Build history of the part. All positions in model axes, mm. Face numbers are marked on the shaded views. A direction names the side the tool comes from. Round coordinates to 2 decimals unless told otherwise and drop trailing zeros. Order: outer loops, then holes, each group sorted by start corner. A loop starts at its lowest first (then second) coordinate and runs counter-clockwise, first axis right, second up. Notation, with made-up numbers: (34.5, -13.75) -> (46.5, -13.75) arc R6 cw to (46.5, -3.75) -> close; hole circle Ø5 at (85.5, 25.25). An arc over 180 degrees is marked (long way). Answer as a JSON object with one key per item and string values.
from build123d import *

# Parameters (mm, degrees)
BRIDA_BASE1_DEPTH          = 89.15
CORTAR_EXTRUIR3_DEPTH      = 100.859660931
CORTAR_EXTRUIR3_DEPTH_BACK = 100.859660931
CROQUIS7_W                 = 3
CROQUIS7_H                 = 17.495
REDONDEO6_R                = 1
REDONDEO8_RADIUS           = 7.11
REDONDEO8_LENGTH           = 3.175
REDONDEO9_RADIUS           = 7.11
REDONDEO9_LENGTH           = 3.175
CORTAR_EXTRUIR4_DEPTH      = 100.859660931
CORTAR_EXTRUIR4_DEPTH_BACK = 100.859660931
CROQUIS14_R                = 1.5
CORTAR_EXTRUIR5_DEPTH      = 99.89399947
CORTAR_EXTRUIR5_DEPTH_BACK = 99.89399947
CROQUIS15_W                = 3.24
CROQUIS15_H                = 30.48


# Sheet-metal steps are written as plain solids
with BuildPart() as part:
    # Croquis1 → Brida base1 (new body)
    with BuildSketch(Plane.XY):
        with BuildLine():
            Line((25.4625, 0), (25.4625, 27.9034))
            ThreePointArc((25.4625, 27.9034), (25.246754855, 28.424254855), (24.7259, 28.64))
            Line((24.7259, 28.64), (0.7366, 28.64))
            ThreePointArc((0.7366, 28.64), (0.215745145, 28.424254855), (0, 27.9034))
            Line((0, 27.9034), (0, 0))
            Line((0, 0), (-3.175, 0))
            Line((-3.175, 0), (-3.175, 27.9034))
            ThreePointArc((-3.175, 27.9034), (-2.029318885, 30.669318885), (0.7366, 31.815))
            Line((0.7366, 31.815), (24.7259, 31.815))
            ThreePointArc((24.7259, 31.815), (27.491818885, 30.669318885), (28.6375, 27.9034))
            Line((28.6375, 27.9034), (28.6375, 0))
            Line((28.6375, 0), (25.4625, 0))
        make_face()
    extrude(amount=BRIDA_BASE1_DEPTH)

    # Croquis7 → Cortar-Extruir3 (cut, two sides: drawn at the far end of the back side and taken through both)
    with BuildSketch(Plane(origin=(28.6375, 0, 0), x_dir=(0, 0, -1), z_dir=(1, 0, 0)).offset(-CORTAR_EXTRUIR3_DEPTH_BACK)):
        with BuildLine():
            Line((0, 31.815), (-51.6, 31.815))
            Line((-51.6, 31.815), (-51.6, 18.22))
            ThreePointArc((-51.6, 18.22), (-50.428427125, 15.391572875), (-47.6, 14.22))
            Line((-47.6, 14.22), (0, 14.22))
            Line((0, 14.22), (0, 31.815))
        make_face()
        with Locations((-87.65, 8.7475)):
            Rectangle(CROQUIS7_W, CROQUIS7_H)
    extrude(amount=CORTAR_EXTRUIR3_DEPTH + CORTAR_EXTRUIR3_DEPTH_BACK, mode=Mode.SUBTRACT)

    # Redondeo6
    redondeo6_edges = [part.edges().sort_by_distance(p)[0] for p in [
        (-1.5875, 17.495, 86.15),
        (-1.5875, 17.495, 89.15),
        (-1.5875, 0, 86.15),
        (27.05, 17.495, 86.15),
        (27.05, 0, 86.15),
        (27.05, 17.495, 89.15),
    ]]
    fillet(redondeo6_edges, radius=REDONDEO6_R)

    # Redondeo8: full round fillet: the end face becomes a half cylinder, R = half its width
    redondeo8_face = Plane((27.05, 7.11, 0), x_dir=(-1, 0, 0), z_dir=(0, 0, -1))  # on the end face: x along it, z out of the body
    redondeo8_slab = redondeo8_face.offset(-REDONDEO8_RADIUS / 2) * Box(REDONDEO8_LENGTH, 2 * REDONDEO8_RADIUS, REDONDEO8_RADIUS, mode=Mode.PRIVATE)  # the body's end, R deep
    redondeo8_round = Plane((27.05, 7.11, 7.11), x_dir=(0, 0, -1), z_dir=(-1, 0, 0)) * Cylinder(REDONDEO8_RADIUS, REDONDEO8_LENGTH, mode=Mode.PRIVATE)  # its axis R under the face
    add(redondeo8_slab - redondeo8_round, mode=Mode.SUBTRACT)

    # Redondeo9: full round fillet: the end face becomes a half cylinder, R = half its width
    redondeo9_face = Plane((-1.5875, 7.11, 0), x_dir=(-1, 0, 0), z_dir=(0, 0, -1))  # on the end face: x along it, z out of the body
    redondeo9_slab = redondeo9_face.offset(-REDONDEO9_RADIUS / 2) * Box(REDONDEO9_LENGTH, 2 * REDONDEO9_RADIUS, REDONDEO9_RADIUS, mode=Mode.PRIVATE)  # the body's end, R deep
    redondeo9_round = Plane((-1.5875, 7.11, 7.11), x_dir=(0, 0, -1), z_dir=(-1, 0, 0)) * Cylinder(REDONDEO9_RADIUS, REDONDEO9_LENGTH, mode=Mode.PRIVATE)  # its axis R under the face
    add(redondeo9_slab - redondeo9_round, mode=Mode.SUBTRACT)

    # Croquis14 → Cortar-Extruir4 (cut, two sides: drawn at the far end of the back side and taken through both)
    with BuildSketch(Plane(origin=(28.6375, 0, 0), x_dir=(0, 0, -1), z_dir=(1, 0, 0)).offset(-CORTAR_EXTRUIR4_DEPTH_BACK)):
        with Locations((-7.11, 7.11)):
            Circle(CROQUIS14_R)
    extrude(amount=CORTAR_EXTRUIR4_DEPTH + CORTAR_EXTRUIR4_DEPTH_BACK, mode=Mode.SUBTRACT)

    # Croquis15 → Cortar-Extruir5 (cut, two sides: drawn at the far end of the back side and taken through both)
    with BuildSketch(Plane(origin=(0, 31.815, 0), x_dir=(1, 0, 0), z_dir=(0, 1, 0)).offset(-CORTAR_EXTRUIR5_DEPTH_BACK)):
        with Locations((12.73125, -70.375)):
            Rectangle(CROQUIS15_W, CROQUIS15_H)
    extrude(amount=CORTAR_EXTRUIR5_DEPTH + CORTAR_EXTRUIR5_DEPTH_BACK, mode=Mode.SUBTRACT)


solid = part.part
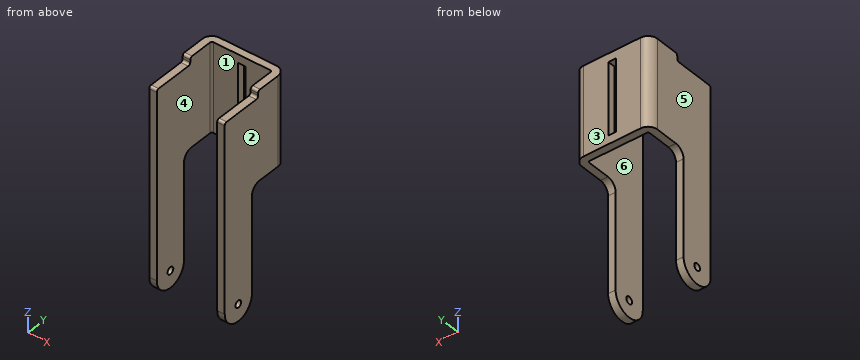
1) Cut at D-D, the plane x = 19. Give the cut face in (y, z) (3 decimals).
Checked values:
{"outline": "(28.64, 51.6) -> (31.815, 51.6) -> (31.815, 89.15) -> (28.64, 89.15) -> close"}
2) Cut at B-B, the plane z = 24. Give the cut face in (x, y) (1 decimal), plus the area to 3 significant figures.
Checked values:
{"outline": "(-3.2, 0) -> (0, 0) -> (0, 14.2) -> (-3.2, 14.2) -> close; (25.5, 0) -> (28.6, 0) -> (28.6, 14.2) -> (25.5, 14.2) -> close", "area": "90.3 mm²"}
3) Pull direction X, two halves, no side cores. Call the marked faces 1, 2, 3 and 4: pulls with the +X half, pulls with the -X half, needs draft (parallel to the pull), parting line crosses it, or undercut.
Checked values:
{"face 1": "undercut", "face 2": "pulls with the +X half", "face 3": "needs draft", "face 4": "undercut"}
4) Which spindle directions (+Z, -Z, +X, -X, +Y, -Y) get a long thin tool onto all of the face, cutting with end or side? Do the marked faces 5 and 6. Say none if no direction does.
Checked values:
{"face 5": "+Z, -Z, -X, +Y, -Y", "face 6": "+Z, -Z, -Y"}
5) Flat gauge pins, fed straight in: pin 1 Ø2.5 at (x, y) = (-1, 9) entering from +Z; pin 2 Ø1.6 at (y, z) = (30, 70) entering from -X; pin 3 Ø3.5 at (y, z) = (31, 72) entering from +X. Where does each tip first touch, or does it go through?
Checked values:
{"pin 1": "stops at z = 86.15", "pin 2": "stops at x = -2.95", "pin 3": "stops at x = 28.4"}
6) Probe L1, parallel to X at y = 20, z = 74 (1 decimal); L2, parallel to Y at x = -2.2, z = 7.11; L3, parallel to Z at x = 27, y = 7.11. List the from-to ranges inside material, lowest first. Write a range as from..to.
Checked values:
{"L1": "x = -3.2..0, 25.5..28.6", "L2": "y = 0..5.61, 8.61..14.22", "L3": "z = 0..5.61, 8.61..86.15"}
7) Cut at C-C, the plane y = 7.11. Count the separate pieces of the cut face and the enclosed holes in it, plus the area to 3 significant figures.
Checked values:
{"separate pieces": "4", "enclosed holes": "0", "area": "528 mm²"}
